For this review, take the finished solid that the model builds, in its own axes (mm). A direction names the side the tool comes from. Round coordinates to 2 decimals unless told otherwise and drop trailing zeros. Order: outer loops, then holes, each group sorted by start corner. A loop starts at its lowest first (then second) coordinate and runs counter-clockwise, first axis right, second up. Notation, with made-up numbers: M 1.25,74 L 42.25,74 A13 ccw 42.25,81 Z; hole C 22.5,46 d1. An arc over 180 degrees is marked long. Answer in a Markdown table with one row per item. Add a question column.
```python
from build123d import *

# Parameters (mm, degrees)
PROFILE_SKETCH_R      = 2.1
PROFILE_EXTRUDE_DEPTH = 125


with BuildPart() as part:
    # Profile Sketch → Profile Extrude (new body)
    with BuildSketch(Plane(origin=(0, 0, 0), x_dir=(0, 0, -1), z_dir=(1, 0, 0))):
        with BuildLine():
            Line((5.42, 10), (-5.42, 10))
            Line((-5.42, 10), (-6.875, 8.545))
            Line((-6.875, 8.545), (-6.875, 8.2))
            Line((-6.875, 8.2), (-4.5, 8.2))
            Line((-4.5, 8.2), (-4.5, 6.56))
            Line((-4.5, 6.56), (-7.16, 3.9))
            Line((-7.16, 3.9), (-9.79, 3.9))
            Line((-9.79, 3.9), (-10, 3.69))
            Line((-10, 3.69), (-10.21, 3.9))
            Line((-10.21, 3.9), (-12.84, 3.9))
            Line((-12.84, 3.9), (-15.5, 6.56))
            Line((-15.5, 6.56), (-15.5, 8.2))
            Line((-15.5, 8.2), (-13.125, 8.2))
            Line((-13.125, 8.2), (-13.125, 8.545))
            Line((-13.125, 8.545), (-14.58, 10))
            Line((-14.58, 10), (-19.5, 10))
            ThreePointArc((-19.5, 10), (-19.853553391, 9.853553391), (-20, 9.5))
            Line((-20, 9.5), (-20, 4.58))
            Line((-20, 4.58), (-18.545, 3.125))
            Line((-18.545, 3.125), (-18.2, 3.125))
            Line((-18.2, 3.125), (-18.2, 5.5))
            Line((-18.2, 5.5), (-16.56, 5.5))
            Line((-16.56, 5.5), (-13.9, 2.838679656))
            Line((-13.9, 2.838679656), (-13.9, 0.21))
            Line((-13.9, 0.21), (-13.69, 0))
            Line((-13.69, 0), (-13.9, -0.21))
            Line((-13.9, -0.21), (-13.9, -2.838679656))
            Line((-13.9, -2.838679656), (-16.56, -5.5))
            Line((-16.56, -5.5), (-18.2, -5.5))
            Line((-18.2, -5.5), (-18.2, -3.125))
            Line((-18.2, -3.125), (-18.545, -3.125))
            Line((-18.545, -3.125), (-20, -4.58))
            Line((-20, -4.58), (-20, -9.5))
            ThreePointArc((-20, -9.5), (-19.853553391, -9.853553391), (-19.5, -10))
            Line((-19.5, -10), (-14.58, -10))
            Line((-14.58, -10), (-13.125, -8.545))
            Line((-13.125, -8.545), (-13.125, -8.2))
            Line((-13.125, -8.2), (-15.5, -8.2))
            Line((-15.5, -8.2), (-15.5, -6.56))
            Line((-15.5, -6.56), (-12.84, -3.9))
            Line((-12.84, -3.9), (-10.21, -3.9))
            Line((-10.21, -3.9), (-10, -3.69))
            Line((-10, -3.69), (-9.79, -3.9))
            Line((-9.79, -3.9), (-7.16, -3.9))
            Line((-7.16, -3.9), (-4.5, -6.56))
            Line((-4.5, -6.56), (-4.5, -8.2))
            Line((-4.5, -8.2), (-6.875, -8.2))
            Line((-6.875, -8.2), (-6.875, -8.545))
            Line((-6.875, -8.545), (-5.42, -10))
            Line((-5.42, -10), (5.42, -10))
            Line((5.42, -10), (6.875, -8.545))
            Line((6.875, -8.545), (6.875, -8.2))
            Line((6.875, -8.2), (4.5, -8.2))
            Line((4.5, -8.2), (4.5, -6.56))
            Line((4.5, -6.56), (7.16, -3.9))
            Line((7.16, -3.9), (9.79, -3.9))
            Line((9.79, -3.9), (10, -3.69))
            Line((10, -3.69), (10.21, -3.9))
            Line((10.21, -3.9), (12.84, -3.9))
            Line((12.84, -3.9), (15.5, -6.56))
            Line((15.5, -6.56), (15.5, -8.2))
            Line((15.5, -8.2), (13.125, -8.2))
            Line((13.125, -8.2), (13.125, -8.545))
            Line((13.125, -8.545), (14.58, -10))
            Line((14.58, -10), (19.5, -10))
            ThreePointArc((19.5, -10), (19.853553391, -9.853553391), (20, -9.5))
            Line((20, -9.5), (20, -4.58))
            Line((20, -4.58), (18.545, -3.125))
            Line((18.545, -3.125), (18.2, -3.125))
            Line((18.2, -3.125), (18.2, -5.5))
            Line((18.2, -5.5), (16.56, -5.5))
            Line((16.56, -5.5), (13.9, -2.838679656))
            Line((13.9, -2.838679656), (13.9, -0.21))
            Line((13.9, -0.21), (13.69, 0))
            Line((13.69, 0), (13.9, 0.21))
            Line((13.9, 0.21), (13.9, 2.838679656))
            Line((13.9, 2.838679656), (16.56, 5.5))
            Line((16.56, 5.5), (18.2, 5.5))
            Line((18.2, 5.5), (18.2, 3.125))
            Line((18.2, 3.125), (18.545, 3.125))
            Line((18.545, 3.125), (20, 4.58))
            Line((20, 4.58), (20, 9.5))
            ThreePointArc((20, 9.5), (19.853553391, 9.853553391), (19.5, 10))
            Line((19.5, 10), (14.58, 10))
            Line((14.58, 10), (13.125, 8.545))
            Line((13.125, 8.545), (13.125, 8.2))
            Line((13.125, 8.2), (15.5, 8.2))
            Line((15.5, 8.2), (15.5, 6.56))
            Line((15.5, 6.56), (12.84, 3.9))
            Line((12.84, 3.9), (10.21, 3.9))
            Line((10.21, 3.9), (10, 3.69))
            Line((10, 3.69), (9.79, 3.9))
            Line((9.79, 3.9), (7.16, 3.9))
            Line((7.16, 3.9), (4.5, 6.56))
            Line((4.5, 6.56), (4.5, 8.2))
            Line((4.5, 8.2), (6.875, 8.2))
            Line((6.875, 8.2), (6.875, 8.545))
            Line((6.875, 8.545), (5.42, 10))
        make_face()
        with Locations((-10, 0)):
            Circle(PROFILE_SKETCH_R, mode=Mode.SUBTRACT)
        with Locations((10, 0)):
            Circle(PROFILE_SKETCH_R, mode=Mode.SUBTRACT)
        Polygon((2.7, 8.2), (-2.7, 8.2), (-2.7, 6.238679656), (-6.1, 2.838679656), (-6.1, -0.21), (-6.1, -2.838679656), (-2.7, -6.238679656), (-2.7, -8.2), (2.7, -8.2), (2.7, -6.238679656), (6.1, -2.838679656), (6.1, -0.21), (6.1, 2.838679656), (2.7, 6.238679656), align=None, mode=Mode.SUBTRACT)
    extrude(amount=PROFILE_EXTRUDE_DEPTH)


solid = part.part
```
1. The part is to be moulded in two halves that separate along Y. For faces 6 (the flat face through (0, 5, 5)), 7 (the flat face through (62, 0, 6.1)), 8 (the flat face through (62, -3.9, 8)), say which applies: pulls with the +Y half, pulls with the -Y half, needs draft (parallel to the pull), parting line crosses it, or undercut.
2. Consider section B-B on x = 34.5. State how many separate pieces and enclosed holes the cut face has, plus the area to 3 significant figures.
3. Consider section A-A on z = 0. Write out the cut boundary in (x, y).
4. Clearance check with flat-ended pins moving along their axes: pin 1 Ø3 at (x, y) = (79.5, -2) entering from -Z; pin 2 Ø1 at (x, z) = (53, 9.5) entering from +Y; pin 3 Ø3 at (x, z) = (92, -11.5) entering from +Y. State where each tip first meets the part, or that it passes through.
5. For faces 1 (the flat face through (62, 3.9, -8)), 2 (the flat face through (62, 2, -13.9)), 3 (the flat face through (62, -10, 17)), 4 (the flat face through (62, 7, -20)), 5 (the flat face through (62, -8.2, 6)), list the 3-axis set-ups (+Z, -Z, +X, -X, +Y, -Y) from which the entire face can be reached by the end or side of a thin tool; tool diameter is ignored.
6. To check wall thickness, follow probe 1 along Z at (x, y) = (68, -0.25); probe 2 along Z at (x, y) = (50, 7.5); probe 3 along Z at (x, y) = (24, -2.5). State the ranges of each line that lie inside material, in increasing order. Write a range as [from, to].
Solved:
| question | item | result |
|---|---|---|
| 1 | face 6 | needs draft |
| 1 | face 7 | undercut |
| 1 | face 8 | pulls with the -Y half |
| 2 | separate pieces | 1 |
| 2 | enclosed holes | 3 |
| 2 | area | 300 mm^2 |
| 3 | outline | M 0,-10 L 125,-10 L 125,-8.2 L 0,-8.2 Z; M 0,8.2 L 125,8.2 L 125,10 L 0,10 Z |
| 4 | pin 1 | stops at z = -18.92 |
| 4 | pin 2 | stops at y = 3.9 |
| 4 | pin 3 | stops at y = 4.06 |
| 5 | face 1 | +X, -X, +Y |
| 5 | face 2 | -Z, +X, -X |
| 5 | face 3 | +Z, -Z, +X, -X, -Y |
| 5 | face 4 | -Z, +X, -X, +Y, -Y |
| 5 | face 5 | +X, -X |
| 6 | probe 1 | z = [-13.9, -12.09], [-7.91, -6.1], [6.1, 7.91], [12.09, 13.9] |
| 6 | probe 2 | z = [-20, -15.5], [-4.5, -2.7], [2.7, 4.5], [15.5, 20] |
| 6 | probe 3 | z = [-13.9, -6.1], [6.1, 13.9] |
